```python
from build123d import *

# Parameters (mm, degrees)
ESQUISSE2_W             = 47.2
ESQUISSE2_H             = 18.3
BOSS_EXTRU_3_DEPTH      = 30
ENL_V_MAT_EXTRU_1_DEPTH = 5
ESQUISSE6_R             = 3.05
ENL_V_MAT_EXTRU_2_DEPTH = 29
CONG_1_R                = 3
ESQUISSE7_W             = 56.209091813
ESQUISSE7_H             = 35.087501562
ENL_V_MAT_EXTRU_3_DEPTH = 10


with BuildPart() as part:
    # Esquisse2 → Boss.-Extru.3 (new body)
    with BuildSketch(Plane.XY):
        with Locations((32.341918096, 14.118251)):
            Rectangle(ESQUISSE2_W, ESQUISSE2_H)
    extrude(amount=BOSS_EXTRU_3_DEPTH)

    # Esquisse3 → Enlèv. mat.-Extru.1 (cut)
    with BuildSketch(Plane(origin=(0, 23.268251, 0), x_dir=(1, 0, 0), z_dir=(0, 1, 0))):
        Polygon((38.115420787, -8.1), (35.228669442, -3.1), (29.45516675, -3.1), (26.568415404, -8.1), (29.45516675, -13.1), (35.228669442, -13.1), align=None)
        Polygon((38.115420787, -21.9), (35.228669442, -16.9), (29.45516675, -16.9), (26.568415404, -21.9), (29.45516675, -26.9), (35.228669442, -26.9), align=None)
    extrude(amount=-ENL_V_MAT_EXTRU_1_DEPTH, mode=Mode.SUBTRACT)

    # Esquisse6 → Enlèv. mat.-Extru.2 (cut)
    with BuildSketch(Plane(origin=(0, 23.268251, 0), x_dir=(1, 0, 0), z_dir=(0, 1, 0))):
        with Locations(Location((32.341903964, -8.100016153, 0), (0, 0, 270))):
            Circle(ESQUISSE6_R)
        with Locations(Location((32.341903964, -21.95, 0), (0, 0, 270))):
            Circle(ESQUISSE6_R)
    extrude(amount=-ENL_V_MAT_EXTRU_2_DEPTH, mode=Mode.SUBTRACT)

    # Congé1
    cong_1_edges = [part.edges().sort_by_distance(p)[0] for p in [
        (55.941918096, 14.118251, 30),
        (8.741918096, 14.118251, 30),
        (55.941918096, 14.118251, 0),
        (8.741918096, 14.118251, 0),
    ]]
    fillet(cong_1_edges, radius=CONG_1_R)

    # Esquisse7 → Enlèv. mat.-Extru.3 (cut)
    with BuildSketch(Plane.XZ.offset(-4.968251)):
        with Locations((35.574310997, 14.252533976)):
            Rectangle(ESQUISSE7_W, ESQUISSE7_H)
    extrude(amount=-ENL_V_MAT_EXTRU_3_DEPTH, mode=Mode.SUBTRACT)


solid = part.part
```
Part model, mm, in its own coordinate system. A direction names the side the tool comes from. Round coordinates to 2 decimals unless told otherwise and drop trailing zeros. Order: outer loops, then holes, each group sorted by start corner. A loop starts at its lowest first (then second) coordinate and runs counter-clockwise, first axis right, second up. Notation, with made-up numbers: M -36.5,-39 L 3.5,-39 A36 ccw 3.5,-3 Z; hole C 15,75.5 d3. An arc over 180 degrees is marked long. Answer in a Markdown table with one row per item. Add a question column.
Q1. Pin check, flat tips, straight feed: pin 1 (8 mm diameter, centred on x = 32.34, z = 21.95, fed in from +Y); pin 2 (5 mm diameter, centred on x = 32.5, z = 8.5, fed in from +Y). Stop position of each tip, or through.
Q2. Cut at D-D on z = 25.5. Give the cut face in (x, y).
Q3. Wall check: L1, parallel to Z at x = 34, y = 20.5; L2, parallel to Z at x = 35, y = 17.5; L3, parallel to X at y = 17.45, z = 21.95. Give the ranges that are in metal, low to high. Write a range as from..to.
Q4. Cut at B-B on z = 6.25. Give the cut face in (x, y), and give its area (3 significant figures).
Q5. Cut at A-A on y = 19.25. Give the cut face in (x, z).
Q6. Cut at C-C on x = 37. Give the cut face in (y, z), and give its area (3 significant figures).
Q7. Mould opens along X. For faces 1 (the face through (27.99, 20.8, 24.36)), 2 (the face through (32, 19, 0)), 3 (the face through (9.6, 19.2, 0.9)) say: +X half, -X half, draft (parallel to the pull), parting line (faces both ways), or undercut.
Q8. 3-axis set-ups, long thin cutter, end or side, ignore diameter. For faces 4 (the face through (32, 14.968, 15)), 5 (the face through (28.032, 20.803, 19.365)): which of +Z, -Z, +X, -X, +Y, -Y reach the whole face in a straight line?
Established:
| question | item | result |
|---|---|---|
| 1 | pin 1 | stops at y = 18.27 |
| 1 | pin 2 | passes through |
| 2 | outline | M 8.74,14.97 L 55.94,14.97 L 55.94,23.27 L 36.04,23.27 L 36.04,18.27 L 28.65,18.27 L 28.65,23.27 L 8.74,23.27 Z |
| 3 | L1 | z = 0..3.1, 13.1..16.9, 26.9..30 |
| 3 | L2 | z = 0..6.6, 9.6..20.45, 23.45..30 |
| 3 | L3 | x = 8.74..29.29, 35.39..55.94 |
| 4 | outline | M 8.74,14.97 L 29.92,14.97 L 29.92,18.27 L 27.64,18.27 L 27.64,23.27 L 8.74,23.27 Z; M 34.77,14.97 L 55.94,14.97 L 55.94,23.27 L 37.05,23.27 L 37.05,18.27 L 34.77,18.27 Z |
| 4 | area | 329 mm2 |
| 5 | outline | M 8.74,3 A3 ccw 11.74,0 L 52.94,0 A3 ccw 55.94,3 L 55.94,27 A3 ccw 52.94,30 L 11.74,30 A3 ccw 8.74,27 Z; hole M 26.57,8.1 L 29.46,3.1 L 35.23,3.1 L 38.12,8.1 L 35.23,13.1 L 29.46,13.1 Z; hole M 26.57,21.9 L 29.46,16.9 L 35.23,16.9 L 38.12,21.9 L 35.23,26.9 L 29.46,26.9 Z |
| 6 | outline | M 14.97,0 L 23.27,0 L 23.27,6.17 L 18.27,6.17 L 18.27,10.03 L 23.27,10.03 L 23.27,19.97 L 18.27,19.97 L 18.27,23.83 L 23.27,23.83 L 23.27,30 L 14.97,30 Z |
| 6 | area | 210 mm2 |
| 7 | face 1 | undercut |
| 7 | face 2 | draft |
| 7 | face 3 | -X half |
| 8 | face 4 | +Z, -Z, +X, -X, -Y |
| 8 | face 5 | +Y |
